from build123d import *

# Parameters (mm, degrees)
SKETCH1_R           = 31.5
BOSS_EXTRUDE1_DEPTH = 70
SKETCH2_R           = 5
BOSS_EXTRUDE2_DEPTH = 44
SKETCH5_R           = 2
CUT_EXTRUDE2_DEPTH  = 10
SKETCH6_R           = 2
CUT_EXTRUDE3_DEPTH  = 5
CIRPATTERN1_COUNT   = 4
CIRPATTERN2_COUNT   = 4


with BuildPart() as part:
    # Sketch1 → Boss-Extrude1 (new body)
    with BuildSketch(Plane.XY):
        Circle(SKETCH1_R)
    extrude(amount=-BOSS_EXTRUDE1_DEPTH)

    # Sketch2 → Boss-Extrude2 (add)
    with BuildSketch(Plane.XY):
        Circle(SKETCH2_R)
    extrude(amount=BOSS_EXTRUDE2_DEPTH)

    # Sketch5 → Cut-Extrude2 (cut)
    with BuildSketch(Plane(origin=(0, 0, -70), x_dir=(-1, 0, 0), z_dir=(0, 0, -1))):
        with Locations((-11, 0)):
            Circle(SKETCH5_R)
    cut_extrude2 = extrude(amount=-CUT_EXTRUDE2_DEPTH, mode=Mode.SUBTRACT)

    # Sketch6 → Cut-Extrude3 (cut)
    with BuildSketch(Plane.XY):
        with Locations((0, 15)):
            Circle(SKETCH6_R)
        with Locations((0, 22)):
            Circle(SKETCH6_R)
    cut_extrude3 = extrude(amount=-CUT_EXTRUDE3_DEPTH, mode=Mode.SUBTRACT)

    # CirPattern1: Cut-Extrude3 ×4 about axis
    cirpattern1_axis = Axis((0, 0, 0), (0, 0, 1))
    for i in range(1, CIRPATTERN1_COUNT):
        add(cut_extrude3.rotate(cirpattern1_axis, i * 360 / CIRPATTERN1_COUNT), mode=Mode.SUBTRACT)

    # CirPattern2: Cut-Extrude2 ×4 about axis
    cirpattern2_axis = Axis((0, 0, 0), (0, 0, 1))
    for i in range(1, CIRPATTERN2_COUNT):
        add(cut_extrude2.rotate(cirpattern2_axis, i * 360 / CIRPATTERN2_COUNT), mode=Mode.SUBTRACT)


solid = part.part
Input: part model. Units: mm. Frame: model coordinates. A direction names the side the tool comes from. Coordinates: 2 decimals unless noted, no trailing zeros. Loops run counter-clockwise (first coordinate to the right, second up) from the corner with the lowest first, then second, coordinate; pieces in that order, holes last. Notation, with made-up numbers: (71.25, -23.5) -> (110.25, -23.5) arc R10 ccw to (110.25, -16.5) -> close; hole circle Ø8 at (29.25, 76.5). An arc over 180 degrees is marked (long way). Write each question's results on one line, items separated by ' | '. Start each with the question number.
Q1. Section C-C, the plane z = 22. Return the cut outline in (x, y), plus the area to 3 significant figures.
Q2. Ray query, line 1 (Y direction, x = 0, z = -1.55); line 2 (Y direction, x = -15, z = -3); line 3 (Z direction, x = 26.5, y = 4). Return the intervals inside material, ascending. Write a range as from..to.
Q3. Pin query (flat end, axial travel): pin 1 (1.5 mm diameter, centred on x = 8, z = -36, fed in from -Y); pin 2 (3.5 mm diameter, centred on x = 0, y = -11, fed in from +Z); pin 3 (6 mm diameter, centred on x = 6, z = 24.5, fed in from +Y). Return the tip coordinate at first contact, or that it passes through.
Q4. Pull-direction query (X, two-part tool) for faces 1 (the flat face through (-11, 0, -60)), 2 (the cylindrical face through (-1.08, -4.88, 21.69)), 3 (the flat face through (0, 0, -70)); classes: released by +X, released by -X, zero draft, split by the parting line, or undercut.
Q5. Section D-D, the plane y = 11. Return the cut outline in (x, z), plus the area to 3 significant figures.
Q6. Reachability of faces 4 (the flat face through (0, -15, -5)), 5 (the cylindrical face through (12.6, -1.2, -65.1)), 6 (the flat face through (0, 0, 44)) from +Z, -Z, +X, -X, +Y, -Y: full face, straight path, thin tool, end or side. Return the list, or none.
Found:
1) outline: circle Ø10 at (0, 0) | area: 78.5 mm2
2) line 1: -31.5..-24, -20..-17, -13..13, 17..20, 24..31.5 | line 2: -27.7..-2, 2..27.7 | line 3: -70..0
3) pin 1: y = -30.65 | pin 2: z = 0 | pin 3: y = 4
4) face 1: undercut | face 2: split by the parting line | face 3: zero draft
5) outline: (-29.52, -70) -> (-2, -70) -> (-2, -60) -> (2, -60) -> (2, -70) -> (29.52, -70) -> (29.52, 0) -> (-29.52, 0) -> close | area: 4,090 mm2
6) face 4: +Z | face 5: -Z | face 6: +Z, +X, -X, +Y, -Y
